Part model, mm, in its own coordinate system. A direction names the side the tool comes from. Coordinates: 2 decimals unless noted, no trailing zeros. Order: outer loops, then holes, each group sorted by start corner. A loop starts at its lowest first (then second) coordinate and runs counter-clockwise, first axis right, second up.
from build123d import *

# Parameters (mm, degrees)
SKETCH_1_R      = 1
EXTRUDE_1_DEPTH = 3


with BuildPart() as part:
    # 草图1 → 凸台-拉伸1 (new body)
    with BuildSketch(Plane.XY):
        with BuildLine():
            Line((-334.183039587, 54.017725717), (-334.183039587, 90.617725717))
            ThreePointArc((-334.183039587, 90.617725717), (-337.363809396, 94.692179032), (-342.088358548, 92.595252304))
            Line((-342.088358548, 92.595252304), (-342.882792815, 91.160117477))
            ThreePointArc((-342.882792815, 91.160117477), (-343.106765877, 90.598023292), (-343.183039587, 89.99777657))
            Line((-343.183039587, 89.99777657), (-343.183039587, 55.020224039))
            ThreePointArc((-343.183039587, 55.020224039), (-343.127859797, 54.508542317), (-342.964857766, 54.020389337))
            Line((-342.964857766, 54.020389337), (-342.495395341, 52.995938343))
            ThreePointArc((-342.495395341, 52.995938343), (-342.129192245, 51.728579438), (-341.494878378, 50.571881888))
            ThreePointArc((-341.494878378, 50.571881888), (-340.783039587, 48.317725717), (-341.494878378, 46.063569546))
            ThreePointArc((-341.494878378, 46.063569546), (-342.304535578, 44.424513925), (-342.583039587, 42.617725717))
            Line((-342.583039587, 42.617725717), (-342.583039587, 40.817725717))
            ThreePointArc((-342.583039587, 40.817725717), (-338.383039587, 36.617725717), (-334.183039587, 40.817725717))
            Line((-334.183039587, 40.817725717), (-334.183039587, 42.617725717))
            ThreePointArc((-334.183039587, 42.617725717), (-334.461543596, 44.424513925), (-335.271200796, 46.063569546))
            ThreePointArc((-335.271200796, 46.063569546), (-335.983039587, 48.317725717), (-335.271200796, 50.571881888))
            ThreePointArc((-335.271200796, 50.571881888), (-334.461543596, 52.21093751), (-334.183039587, 54.017725717))
        make_face()
        with Locations((-338.383039587, 84.617725717)):
            Circle(SKETCH_1_R, mode=Mode.SUBTRACT)
        with Locations((-338.383039587, 78.617725717)):
            Circle(SKETCH_1_R, mode=Mode.SUBTRACT)
        with Locations((-338.383039587, 40.817725717)):
            Circle(SKETCH_1_R, mode=Mode.SUBTRACT)
        with Locations((-338.383039587, 63.617725717)):
            Circle(SKETCH_1_R, mode=Mode.SUBTRACT)
        with Locations((-338.383039587, 70.617725717)):
            Circle(SKETCH_1_R, mode=Mode.SUBTRACT)
        with BuildLine():
            Line((-340.183039587, 59.211838267), (-340.183039587, 86.460803779))
            ThreePointArc((-340.183039587, 86.460803779), (-340.783039587, 87.060803779), (-341.383039587, 86.460803779))
            Line((-341.383039587, 86.460803779), (-341.383039587, 55.817725717))
            ThreePointArc((-341.383039587, 55.817725717), (-335.933549844, 54.08567491), (-339.383039587, 58.646152842))
            ThreePointArc((-339.383039587, 58.646152842), (-339.929449749, 58.721940318), (-340.183039587, 59.211838267))
        make_face(mode=Mode.SUBTRACT)
        with BuildLine():
            Line((-339.433039587, 90.617725717), (-339.433039587, 88.915521264))
            ThreePointArc((-339.433039587, 88.915521264), (-336.383039587, 90.617725717), (-339.433039587, 92.31993017))
            Line((-339.433039587, 92.31993017), (-339.433039587, 90.617725717))
        make_face(mode=Mode.SUBTRACT)
    extrude(amount=EXTRUDE_1_DEPTH)


solid = part.part
Q1. Cut at B-B on x = -338. Count the separate pieces of the cut face and the enclosed holes in it, and give its area (3 significant figures).
Results list:
separate pieces: 8
enclosed holes: 0
area: 117 mm2
Q2. Mould opens along X. For faces 1 (the face through (-334.454, 44.4, 1.479)), 2 (the face through (-337.46, 84.23, 1.48)), 3 (the face through (-340.77, 87.06, 1.48)), 4 (the face through (-343.13, 54.52, 1.48)) say: pulls with the +X half, pulls with the -X half, needs draft (parallel to the pull), parting line crosses it, or undercut.
Results list:
face 1: pulls with the +X half
face 2: undercut
face 3: undercut
face 4: pulls with the -X half
Q3. Pin check, flat tips, straight feed: pin 1 Ø0.9 at (y, z) = (91.5, 1.5) entering from +X; pin 2 Ø1.4 at (y, z) = (41.5, 1) entering from -X. Stop position of each tip, or through.
Results list:
pin 1: stops at x = -334.21
pin 2: stops at x = -342.58
Q4. Cut at A-A on y = 68.5. Write the cut outline in (x, z), and give its area (3 significant figures).
Results list:
outline: (-343.18, 0) - (-341.38, 0) - (-341.38, 3) - (-343.18, 3) - close; (-340.18, 0) - (-334.18, 0) - (-334.18, 3) - (-340.18, 3) - close
area: 23.4 mm2
Q5. Wall check: line 1 along X through (y, z) = (73.5, 1.7); line 2 along X through (y, z) = (71.5, 1.8); line 3 along X through (y, z) = (58.5, 1.6). Give the ranges that are in metal, low to high.
Results list:
line 1: x = -343.18 to -341.38, -340.18 to -334.18
line 2: x = -343.18 to -341.38, -340.18 to -338.85, -337.91 to -334.18
line 3: x = -343.18 to -341.38, -337.04 to -334.18
Q6. Which spindle directions (+Z, -Z, +X, -X, +Y, -Y) get a long thin tool onto all of the face, cutting with end or side? Do faces 5 (the face through (-343.183, 73, 1)), 6 (the face through (-342.297, 44.449, 1.479)), 7 (the face through (-342.583, 42, 1)), 8 (the face through (-341.383, 71, 1)), 9 (the face through (-334.47, 52.19, 1.48)). Say none if no direction does.
Results list:
face 5: +Z, -Z, -X, +Y, -Y
face 6: +Z, -Z, -X
face 7: +Z, -Z, -X, -Y
face 8: +Z, -Z
face 9: +Z, -Z, +X
Q7. Cut at D-D on z = 1.35. Write the cut outline in (x, y) (3 decimals), and give its area (3 significant figures).
Results list:
outline: (-343.183, 55.02) arc R2.4 ccw to (-342.965, 54.02) - (-342.495, 52.996) arc R6 ccw to (-341.495, 50.572) arc R3.925 cw to (-341.495, 46.064) arc R6 ccw to (-342.583, 42.618) - (-342.583, 40.818) arc R4.2 ccw to (-334.183, 40.818) - (-334.183, 42.618) arc R6 ccw to (-335.271, 46.064) arc R3.925 cw to (-335.271, 50.572) arc R6 ccw to (-334.183, 54.018) - (-334.183, 90.618) arc R4.2 ccw to (-342.088, 92.595) - (-342.883, 91.16) arc R2.4 ccw to (-343.183, 89.998) - close; hole (-341.383, 55.818) arc R3 ccw (long way) to (-339.383, 58.646) arc R0.6 cw to (-340.183, 59.212) - (-340.183, 86.461) arc R0.6 ccw to (-341.383, 86.461) - close; hole (-339.433, 88.916) arc R2 ccw (long way) to (-339.433, 92.32) - close; hole circle Ø2 at (-338.383, 40.818); hole circle Ø2 at (-338.383, 63.618); hole circle Ø2 at (-338.383, 70.618); hole circle Ø2 at (-338.383, 78.618); hole circle Ø2 at (-338.383, 84.618)
area: 387 mm2
Q8. Cut at C-C on x = -334.75. Write the cut outline in (y, z), and give its area (3 significant figures).
Results list:
outline: (38.71, 0) - (45.16, 0) - (45.16, 3) - (38.71, 3) - close; (51.47, 0) - (92.73, 0) - (92.73, 3) - (51.47, 3) - close
area: 143 mm2
